from build123d import *

# Parameters (mm, degrees)
SKETCH_1_R          = 4.015
EXTRUDE_1_DEPTH     = 50
EXTRUDE_2_DEPTH     = 3
CUT_EXTRUDE_1_DEPTH = 1


with BuildPart() as part:
    # 스케치1 → 보스-돌출1 (new body)
    with BuildSketch(Plane(origin=(0, 0, 0), x_dir=(1, 0, 0), z_dir=(0, 1, 0))):
        Circle(SKETCH_1_R)
    extrude(amount=EXTRUDE_1_DEPTH)

    # 스케치2 → 보스-돌출2 (add)
    with BuildSketch(Plane.XZ):
        Polygon((6.345806764, -15.320132754), (15.320132754, -6.345806764), (15.320132754, 6.345806764), (6.345806764, 15.320132754), (-6.345806764, 15.320132754), (-15.320132754, 6.345806764), (-15.320132754, -6.345806764), (-6.345806764, -15.320132754), align=None)
    extrude(amount=EXTRUDE_2_DEPTH)

    # 스케치3 → 컷-돌출1 (cut)
    with BuildSketch(Plane.XZ.offset(3)):
        Polygon((-14.320132754, -5.931593202), (-5.931593202, -14.320132754), (5.931593202, -14.320132754), (14.320132754, -5.931593202), (14.320132754, 5.931593202), (5.931593202, 14.320132754), (-5.931593202, 14.320132754), (-14.320132754, 5.931593202), align=None)
        Polygon((-5.517379639, -13.320132754), (5.517379639, -13.320132754), (13.320132754, -5.517379639), (13.320132754, 5.517379639), (5.517379639, 13.320132754), (-5.517379639, 13.320132754), (-13.320132754, 5.517379639), (-13.320132754, -5.517379639), align=None, mode=Mode.SUBTRACT)
    extrude(amount=-CUT_EXTRUDE_1_DEPTH, mode=Mode.SUBTRACT)


solid = part.part
Model file for the job. Use its own axes, mm. A direction names the side the tool comes from. Give positions to 0.01 mm unless a question says otherwise; leave off trailing zeros. Order: outer loops, then holes, each group sorted by start corner. A loop starts at its lowest first (then second) coordinate and runs counter-clockwise, first axis right, second up. Notation, with made-up numbers: (12.25, 1) - (55.25, 1) arc R27 cw to (55.25, 21) - close; hole circle Ø3 at (78.25, 36.25). An arc over 180 degrees is marked (long way). Return JSON: item names as keys, results as strings.
1) Pull direction X, two halves, no side cores. Call faces 1 (the flat face through (15, -3, 0)), 2 (the flat face through (-10.07, -2.51, 10.18)), 3 (the flat face through (9.473, -2.507, 9.364)), 4 (the cylindrical face through (-0.52, 24.65, -3.98)): pulls with the +X half, pulls with the -X half, needs draft (parallel to the pull), parting line crosses it, or undercut.
Geometry says:
{"face 1": "needs draft", "face 2": "undercut", "face 3": "undercut", "face 4": "parting line crosses it"}
2) Cut at C-C, the plane y = 11.5. Give the cut face in (x, z) (3 decimals), plus the area to 3 significant figures.
Geometry says:
{"outline": "circle Ø8.03 at (0, 0)", "area": "50.6 mm²"}
3) Cut at A-A, the plane x = 0. Give the cut face in (y, z) (3 decimals), plus the area to 3 significant figures.
Geometry says:
{"outline": "(-3, -15.32) - (0, -15.32) - (0, -4.015) - (50, -4.015) - (50, 4.015) - (0, 4.015) - (0, 15.32) - (-3, 15.32) - (-3, 14.32) - (-2, 14.32) - (-2, 13.32) - (-3, 13.32) - (-3, -13.32) - (-2, -13.32) - (-2, -14.32) - (-3, -14.32) - close", "area": "491 mm²"}
4) Cut at D-D, the plane x = -9. Give the cut face in (y, z), plus the area to 3 significant figures.
Geometry says:
{"outline": "(-3, -12.67) - (0, -12.67) - (0, 12.67) - (-3, 12.67) - (-3, 11.25) - (-2, 11.25) - (-2, 9.84) - (-3, 9.84) - (-3, -9.84) - (-2, -9.84) - (-2, -11.25) - (-3, -11.25) - close", "area": "73.2 mm²"}
5) Probe line 1 (Y direction, x = 3.5, z = -7); line 2 (Z direction, x = -2.5, y = 35); line 3 (X direction, y = 33.5, z = -1.5). List the from-to ranges inside material, lowest first. Write a range as from..to.
Geometry says:
{"line 1": "-3..0", "line 2": "-3.14..3.14", "line 3": "-3.72..3.72"}
6) 3-axis set-ups, long thin cutter, end or side, ignore diameter. For faces 5 (the flat face through (10.07, -2.51, -10.18)), 6 (the flat face through (3, 0, 4)), 7 (the flat face through (10.77, -1.479, -10.896)): which of +Z, -Z, +X, -X, +Y, -Y reach the whole face in a straight line?
Geometry says:
{"face 5": "-Y", "face 6": "+Y", "face 7": "-Z, +X, +Y, -Y"}
7) Cut at B-B, the plane z = 0. Give the cut face in (x, y) (3 decimals).
Geometry says:
{"outline": "(-15.32, -3) - (-14.32, -3) - (-14.32, -2) - (-13.32, -2) - (-13.32, -3) - (13.32, -3) - (13.32, -2) - (14.32, -2) - (14.32, -3) - (15.32, -3) - (15.32, 0) - (4.015, 0) - (4.015, 50) - (-4.015, 50) - (-4.015, 0) - (-15.32, 0) - close"}
8) Flat gauge pins, fed straight in: P1, Ø8, axis at x = -5.5, y = 28, coming from the -Z side; P2, Ø5, axis at x = 2, z = -7, coming from the +Y side; P3, Ø4, axis at y = 10.5, z = -3.5, coming from the +X side. Where does each tip first touch, or does it go through?
Geometry says:
{"P1": "z = -3.72", "P2": "y = 0", "P3": "x = 3.72"}
